from build123d import *

# Parameters (mm, degrees)
EXTRUDE_2_DEPTH     = 3
SKETCH_4_R          = 47.5
CUT_EXTRUDE_1_DEPTH = 3
EXTRUDE_3_DEPTH     = 80
EXTRUDE_7_DEPTH     = 3
EXTRUDE_11_DEPTH    = 3
EXTRUDE_12_DEPTH    = 3
EXTRUDE_13_DEPTH    = 3
EXTRUDE_14_DEPTH    = 3
EXTRUDE_15_DEPTH    = 3
EXTRUDE_16_DEPTH    = 3
EXTRUDE_17_DEPTH    = 3
EXTRUDE_18_DEPTH    = 3
EXTRUDE_19_DEPTH    = 3
EXTRUDE_20_DEPTH    = 3
EXTRUDE_21_DEPTH    = 3


with BuildPart() as part:
    # 草图3 → 凸台-拉伸2 (new body)
    with BuildSketch(Plane(origin=(0, 0, 0), x_dir=(1, 0, 0), z_dir=(0, 1, 0))):
        Polygon((195.4, 0), (97.7, 169.221363899), (-97.7, 169.221363899), (-195.4, 0), (-97.7, -169.221363899), (97.7, -169.221363899), align=None)
    extrude(amount=EXTRUDE_2_DEPTH)

    # 草图4 → 切除-拉伸1 (cut)
    with BuildSketch(Plane(origin=(0, 3, 0), x_dir=(1, 0, 0), z_dir=(0, 1, 0))):
        with Locations(Location((0, 0, 0), (0, 0, 270))):
            Circle(SKETCH_4_R)
    extrude(amount=-CUT_EXTRUDE_1_DEPTH, mode=Mode.SUBTRACT)

    # 草图5 → 凸台-拉伸3 (add)
    with BuildSketch(Plane(origin=(0, 3, 0), x_dir=(1, 0, 0), z_dir=(0, 1, 0))):
        Polygon((83.24, 144.175909222), (-83.24, 144.175909222), (-166.48, 0), (-83.24, -144.175909222), (83.24, -144.175909222), (166.48, 0), align=None)
        Polygon((-80.729537332, 141.005291398), (-162.478933084, 0.588815534), (-81.749395753, -140.416475864), (80.729537332, -141.005291398), (162.478933084, -0.588815534), (81.749395753, 140.416475864), align=None, mode=Mode.SUBTRACT)
    extrude(amount=EXTRUDE_3_DEPTH)

    # 草图11 → 凸台-拉伸7 (add)
    with BuildSketch(Plane(origin=(83.24, 0, 0), x_dir=(0, 0, -1), z_dir=(1, 0, 0))):
        Polygon((144.175909222, 3), (144.175909222, 53), (183.582235223, 53), (169.299378366, 3), align=None)
    extrude(amount=-EXTRUDE_7_DEPTH)

    # 草图15 → 凸台-拉伸11 (add)
    with BuildSketch(Plane(origin=(-41.62, 0, -72.087954611), x_dir=(-0.8660254037844382, 0, 0.500000000000001), z_dir=(-0.500000000000001, 0, -0.8660254037844382))):
        Polygon((-144.175909222, 53), (-144.175909222, 3), (-169.299052365, 3), (-183.581909222, 53), align=None)
    extrude(amount=-EXTRUDE_11_DEPTH)

    # 草图17 → 凸台-拉伸12 (add)
    with BuildSketch(Plane(origin=(-41.62, 0, -72.087954611), x_dir=(-0.8660254037844382, 0, 0.500000000000001), z_dir=(-0.500000000000001, 0, -0.8660254037844382))):
        Polygon((144.175909222, 3), (169.221363899, 3), (183.504220757, 53), (144.175909222, 53), align=None)
    extrude(amount=-EXTRUDE_12_DEPTH)

    # 草图19 → 凸台-拉伸13 (add)
    with BuildSketch(Plane(origin=(83.24, 0, 0), x_dir=(0, 0, -1), z_dir=(1, 0, 0))):
        Polygon((-144.175909222, 3), (-144.175909222, 53), (-183.495909222, 53), (-169.213052365, 3), align=None)
    extrude(amount=-EXTRUDE_13_DEPTH)

    # 草图20 → 凸台-拉伸14 (add)
    with BuildSketch(Plane(origin=(-83.24, 0, 0), x_dir=(0, 0, -1), z_dir=(1, 0, 0))):
        Polygon((144.175909222, 3), (144.175909222, 53), (183.495909222, 53), (169.213052365, 3), align=None)
    extrude(amount=EXTRUDE_14_DEPTH)

    # 草图22 → 凸台-拉伸15 (add)
    with BuildSketch(Plane(origin=(-83.24, 0, 0), x_dir=(0, 0, -1), z_dir=(1, 0, 0))):
        Polygon((-144.175909222, 53), (-144.175909222, 3), (-169.213052365, 3), (-183.495909222, 53), align=None)
    extrude(amount=EXTRUDE_15_DEPTH)

    # 草图23 → 凸台-拉伸16 (add)
    with BuildSketch(Plane(origin=(-41.62, 0, 72.087954611), x_dir=(-0.8660254037844406, 0, -0.4999999999999966), z_dir=(0.4999999999999966, 0, -0.8660254037844406))):
        Polygon((-144.175909222, 53), (-144.175909222, 3), (-169.091328291, 3), (-183.495909222, 52.96506828), align=None)
    extrude(amount=EXTRUDE_16_DEPTH)

    # 草图24 → 凸台-拉伸17 (add)
    with BuildSketch(Plane(origin=(41.62, 0, -72.087954611), x_dir=(-0.866025403784439, 0, -0.4999999999999994), z_dir=(0.4999999999999994, 0, -0.866025403784439))):
        Polygon((-144.175909222, 3), (-169.213052365, 3), (-183.495909222, 53), (-144.175909222, 53), align=None)
    extrude(amount=-EXTRUDE_17_DEPTH)

    # 草图26 → 凸台-拉伸18 (add)
    with BuildSketch(Plane(origin=(-41.62, 0, 72.087954611), x_dir=(-0.8660254037844406, 0, -0.4999999999999966), z_dir=(0.4999999999999966, 0, -0.8660254037844406))):
        Polygon((144.175909222, 53), (144.175909222, 3), (169.213052365, 3), (183.495909222, 53), align=None)
    extrude(amount=EXTRUDE_18_DEPTH)

    # 草图27 → 凸台-拉伸19 (add)
    with BuildSketch(Plane(origin=(41.62, 0, -72.087954611), x_dir=(-0.866025403784439, 0, -0.4999999999999994), z_dir=(0.4999999999999994, 0, -0.866025403784439))):
        Polygon((144.175909222, 53), (144.175909222, 3), (169.137463214, 3), (183.495909222, 52.978345593), align=None)
    extrude(amount=-EXTRUDE_19_DEPTH)

    # 草图28 → 凸台-拉伸20 (add)
    with BuildSketch(Plane(origin=(41.62, 0, 72.087954611), x_dir=(-0.8660254037844407, 0, 0.4999999999999965), z_dir=(-0.4999999999999965, -1.145624345781526e-15, -0.8660254037844407))):
        Polygon((144.175909222, 53), (144.175909222, 3), (169.213052365, 3), (183.495909222, 53), align=None)
    extrude(amount=EXTRUDE_20_DEPTH)

    # 草图31 → 凸台-拉伸21 (add)
    with BuildSketch(Plane(origin=(41.62, 0, 72.087954611), x_dir=(-0.8660254037844407, 0, 0.4999999999999965), z_dir=(-0.4999999999999965, -1.145624345781526e-15, -0.8660254037844407))):
        Polygon((-144.175909222, 53), (-144.175909222, 3), (-169.213052365, 3), (-183.495909222, 53), align=None)
    extrude(amount=EXTRUDE_21_DEPTH)


solid = part.part
Can you work these out from the model? Positions are in its coordinate system, mm. A direction names the side the tool comes from. Round coordinates to 2 decimals unless told otherwise and drop trailing zeros. Write each loop counter-clockwise with the first axis right and the second up, starting at its lowest first coordinate (ties: lowest second). Pieces come first, ordered by that corner, then holes. Notation, with made-up numbers: M 88,11.5 L 93,11.5 A22 ccw 93,41.5 Z; hole C -19.5,-2 d8. An arc over 180 degrees is marked long. Use a Markdown table: item, result.
Item 1: I want a section at A-A (x = 7). List the corners of the cut face in (y, z) for me, and give its area (3 significant figures).
Found:
| item | result |
|---|---|
| outline | M 0,-169.22 L 3,-169.22 L 3,-144.18 L 83,-144.18 L 83,-140.69 L 3,-140.69 L 3,-46.98 L 0,-46.98 Z; M 0,46.98 L 3,46.98 L 3,140.74 L 83,140.74 L 83,144.18 L 3,144.18 L 3,169.22 L 0,169.22 Z |
| area | 1,290 mm2 |
Item 2: For pin 1 Ø0.9 at (x, z) = (-81.5, 155.5) entering from +Y; pin 2 Ø4 at (y, z) = (29, 14.5) entering from -X; pin 3 Ø6 at (y, z) = (10, 20.5) entering from +X, each with a flat end and sliding along its axis, tell me the tip position at first contact or that it passes through.
Found:
| item | result |
|---|---|
| pin 1 | stops at y = 53 |
| pin 2 | stops at x = -194.79 |
| pin 3 | stops at x = 156.38 |
Item 3: If I drill on line 1 along Z through (x, y) = (67.5, 4); line 2 along Z through (x, y) = (104, 29); line 3 along X through (y, z) = (1, 0), over which ranges is the centre line in solid material (lowest first)? Write a range as [from, to].
Found:
| item | result |
|---|---|
| line 1 | z = [-144.18, -140.47], [140.96, 144.18] |
| line 2 | z = [-156.16, -152.7], [-108.22, -101.55], [101.03, 108.22], [152.7, 156.16] |
| line 3 | x = [-195.4, -47.5], [47.5, 195.4] |
Item 4: Which directions (+Z, -Z, +X, -X, +Y, -Y) give clear straight access to the entire face, cutting with the end or side of a thin tool? Please do faces 1 (the face through (83.24, 28, 160)), 2 (the face through (-46.37, 1.52, -10.3)), 3 (the face through (92, 3, -160)), 4 (the face through (103, 3, 115)), 5 (the face through (179.484, 28.35, 7.508)).
Found:
| item | result |
|---|---|
| face 1 | +Z, +Y |
| face 2 | +Y, -Y |
| face 3 | -Z, +Y |
| face 4 | +Y |
| face 5 | +X, +Y |
Item 5: We'd pull the mould along X, two halves only. Please class faces 6 (the face through (-81.761, 27.65, 176.255)), 7 (the face through (-177.99, 28.35, 10.11)), 8 (the face through (111.835, 27.65, -158.977)): released by +X, released by -X, zero draft, split by the parting line, or undercut.
Found:
| item | result |
|---|---|
| face 6 | zero draft |
| face 7 | undercut |
| face 8 | released by +X |
Item 6: I want a section at B-B (x = 130). List the corners of the cut face in (y, z) for me, and give its area (3 significant figures).
Found:
| item | result |
|---|---|
| outline | M 0,-113.28 L 3,-113.28 L 3,-63.19 L 83,-63.19 L 83,-56.14 L 3,-56.14 L 3,56.38 L 83,56.38 L 83,63.19 L 3,63.19 L 3,113.28 L 0,113.28 Z |
| area | 1,790 mm2 |
